The figure shows three views and two pictorial views of one solid part (mm, origin at its lowest corner). Answer the questions. Coordinates: 2 decimals unless noted, no trailing zeros. Loops run counter-clockwise (first coordinate to the right, second up) from the corner with the lowest first, then second, coordinate; pieces in that order, holes last. Notation, with made-up numbers: M 76.5,48 L 135.5,48 A17 ccw 135.5,72 Z; hole C 41,74.5 d3. An arc over 180 degrees is marked long. Write each question's results on one line, items separated by ' | '.
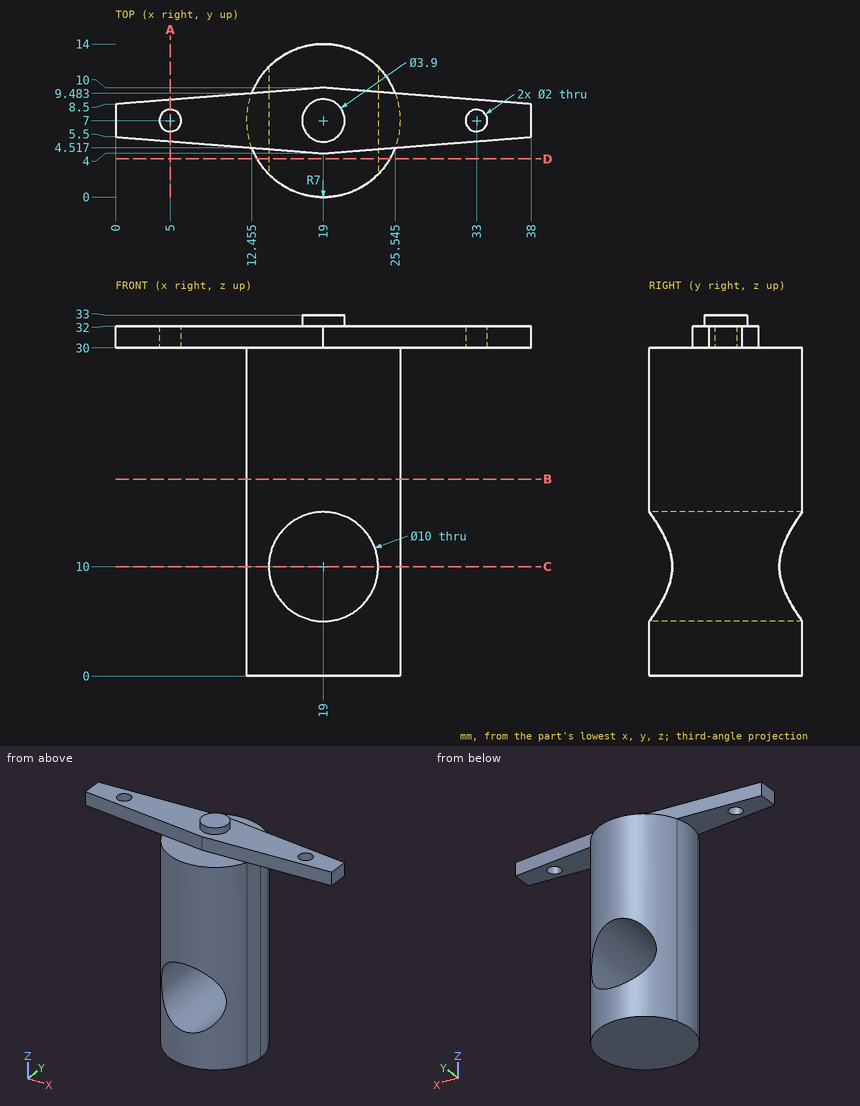
1) Find section A-A, the plane x = 5. Give the vertices of the cut face in (y, z) (1 decimal).
Check result:
outline: M 5.1,30 L 6,30 L 6,32 L 5.1,32 Z; M 8,30 L 8.9,30 L 8.9,32 L 8,32 Z
2) Given pin 1 Ø10 at (x, z) = (15, 12.5) entering from +Y; pin 2 Ø5.5 at (x, y) = (8, 6.5) entering from -Z; pin 3 Ø2 at (y, z) = (3, 23.5) entering from -X (1 decimal); pin 4 Ø2 at (y, z) = (5.5, 26) entering from -X, each flat-ended and moving along its own axis, determine where each tip first touches the part or whether it passes through.
Check result:
pin 1: y = 14 | pin 2: z = 30 | pin 3: x = 12.7 | pin 4: x = 12.02
3) Straight lines are drawn through the part: probe 1 along Z at (x, y) = (19, 11.5); probe 2 along Z at (x, y) = (19, 9.75); probe 3 along Z at (x, y) = (2.5, 5.5). For each, find the intervals that lie inside material, in ascending order. Write a range as [from, to].
Check result:
probe 1: [0, 5], [15, 30] | probe 2: [0, 5], [15, 32] | probe 3: [30, 32]
4) Find section D-D, the plane y = 3.5. Give the vertices of the cut face in (x, z), and give its area (3 significant figures).
Check result:
outline: M 12.94,0 L 25.06,0 L 25.06,30 L 12.94,30 Z; hole C 19,10 d10 | area: 285 mm^2
5) Find section C-C, the plane z = 10. Give the vertices of the cut face in (x, y) (1 decimal), and give its area (3 significant figures).
Check result:
outline: M 14,2.1 L 14,11.9 A7 ccw Z; M 24,2.1 A7 ccw 24,11.9 Z | area: 27.0 mm^2
6) Find section B-B, the plane z = 18. Give the vertices of the cut face in (x, y) (1 decimal), and give its area (3 significant figures).
Check result:
outline: C 19,7 d14 | area: 154 mm^2
